The listing builds one solid part. Answer for the finished solid, in the listing's coordinates (mm). A direction names the side the tool comes from. Give positions to 0.01 mm unless a question says otherwise; leave off trailing zeros. Write each loop counter-clockwise with the first axis right and the second up, starting at its lowest first coordinate (ties: lowest second). Pieces come first, ordered by that corner, then holes. Notation, with made-up numbers: (58, 27.5) - (73, 27.5) arc R11 ccw to (73, 44.5) - close; hole circle Ø8 at (-9, 48.5). An arc over 180 degrees is marked (long way). Return JSON: item names as keys, results as strings.
from build123d import *

# Parameters (mm, degrees)
F1_DEPTH = 25.4
F3_DEPTH = 25.4


with BuildPart() as f1:
    # F0 (on Front) → F1 (new body)
    with BuildSketch(Plane.XZ):
        Polygon((-22.690213, 17.148396), (-22.690213, -46.351604), (28.109787, -46.351604), (15.409787, 17.148396), align=None)
    extrude(amount=F1_DEPTH)

    # F2 (on face) → F3 (join)
    with BuildSketch(Plane(origin=(0, 0, 0), x_dir=(-1, 0, 0), z_dir=(0, 1, 0))):
        Polygon((-66.209787, -46.351604), (-28.109787, -46.351604), (-15.409787, 17.148396), align=None)
        Polygon((-28.109787, -46.351604), (22.690213, -46.351604), (22.690213, 17.148396), (-15.409787, 17.148396), align=None)
    extrude(amount=F3_DEPTH)


solid = f1.part
Item 1: A cutting plane is placed at C-C on x = 24. Determine the outline of the cut face in (y, z).
Answer below:
{"outline": "(-25.4, -46.35) - (25.4, -46.35) - (25.4, 6.41) - (0, 6.41) - (0, -25.8) - (-25.4, -25.8) - close"}
Item 2: For faces 1 (the face through (21.85, -12.52, -15.05)), 2 (the face through (13, 25.4, -21)), determine the directions among +Z, -Z, +X, -X, +Y, -Y from which every point of the face is accessible in a straight line to the end or side of a thin tool.
Answer below:
{"face 1": "+Z, +X, -Y", "face 2": "+Z, -Z, +X, -X, +Y"}
Item 3: Consider L1, parallel to Y at x = 60.5, z = -44; L2, parallel to X at y = -12, z = -30; L3, parallel to X at y = -21, z = 5. Determine where each line is inside the solid, lowest interval first.
Answer below:
{"L1": "y = 0 to 25.4", "L2": "x = -22.69 to 24.84", "L3": "x = -22.69 to 17.84"}
Item 4: A cutting plane is placed at D-D on y = 21. Determine the outline of the cut face in (x, z).
Answer below:
{"outline": "(-22.69, -46.35) - (66.21, -46.35) - (15.41, 17.15) - (-22.69, 17.15) - close"}
Item 5: A cutting plane is placed at B-B on z = -20. Determine the outline of the cut face in (x, y).
Answer below:
{"outline": "(-22.69, -25.4) - (22.84, -25.4) - (22.84, 0) - (45.13, 0) - (45.13, 25.4) - (-22.69, 25.4) - close"}
Item 6: Flat-ended cylindrical pins translate along their axes: P1, Ø10, axis at y = -17, z = -30, coming from the +X side; P2, Ø2, axis at x = 40, y = 0.5, coming from the +Z side; P3, Ø10, axis at y = -10, z = -24, coming from the +X side. Find the tip coordinate at first contact, or state that the pin passes through.
Answer below:
{"P1": "stops at x = 25.84", "P2": "stops at z = -12.34", "P3": "stops at x = 24.64"}
Item 7: A cutting plane is placed at A-A on y = -1.5. Determine the outline of the cut face in (x, z), then the cut area to 3 significant figures.
Answer below:
{"outline": "(-22.69, -46.35) - (28.11, -46.35) - (15.41, 17.15) - (-22.69, 17.15) - close", "area": "2,820 mm²"}
